```python
from build123d import *

# Parameters (mm, degrees)
F0_W     = 272
F0_H     = 60
F0_R     = 2.75
F0_R_2   = 4
F1_DEPTH = 5


with BuildPart() as f1:
    # F0 (on Front) → F1 (new body)
    with BuildSketch(Plane.XZ):
        Rectangle(F0_W, F0_H)
        with Locations((-62, -12.5)):
            Circle(F0_R, mode=Mode.SUBTRACT)
        with Locations((-16, -12.5)):
            Circle(F0_R, mode=Mode.SUBTRACT)
        with Locations((16, -12.5)):
            Circle(F0_R, mode=Mode.SUBTRACT)
        with Locations((62, -12.5)):
            Circle(F0_R, mode=Mode.SUBTRACT)
        with Locations((-119, 0)):
            Circle(F0_R_2, mode=Mode.SUBTRACT)
        with Locations((-95, 0)):
            Circle(F0_R_2, mode=Mode.SUBTRACT)
        with Locations((-62, 12.5)):
            Circle(F0_R, mode=Mode.SUBTRACT)
        with Locations((-16, 12.5)):
            Circle(F0_R, mode=Mode.SUBTRACT)
        with Locations((16, 12.5)):
            Circle(F0_R, mode=Mode.SUBTRACT)
        with Locations((62, 12.5)):
            Circle(F0_R, mode=Mode.SUBTRACT)
        with Locations((95, 0)):
            Circle(F0_R_2, mode=Mode.SUBTRACT)
        with Locations((119, 0)):
            Circle(F0_R_2, mode=Mode.SUBTRACT)
    extrude(amount=F1_DEPTH)


solid = f1.part
```
The listing builds one solid part. Answer for the finished solid, in the listing's coordinates (mm). Give positions to 0.01 mm unless a question says otherwise; leave off trailing zeros. Order: outer loops, then holes, each group sorted by start corner. A loop starts at its lowest first (then second) coordinate and runs counter-clockwise, first axis right, second up. Notation, with made-up numbers: M 6,63 L 59,63 A23 ccw 59,93 Z; hole C 29,31.5 d11. An arc over 180 degrees is marked long. Put each result on its own line as item: value. Start each with the question number.
Item 1: The part is cut by section D-D, the plane y = -3.85. State how many separate pieces and enclosed holes the cut face has, and give its area (3 significant figures).
Item 2: The part is cut by section A-A, the plane z = 0. Determine the outline of the cut face in (x, y).
Item 3: The part is cut by section C-C, the plane x = 119. Determine the outline of the cut face in (y, z).
Item 4: Find the intervals of material crossed by line 1 along Z through (x, y) = (-16, -1.8); line 2 along Z through (x, y) = (-95, -3); line 3 along X through (y, z) = (-2.55, 14.5), in increasing order.
Item 5: For a pull along Z with two mould halves and no side action, classify faces 1 (the face through (-2, -2, -30)), 2 (the face through (91, -2, 0)), 3 (the face through (136, -2, 0)) as +Z half, -Z half, draft (parallel to the pull), parting line (faces both ways), or undercut.
Item 6: The part is cut by section B-B, the plane x = -62. Determine the outline of the cut face in (y, z).
Answer key:
1. separate pieces: 1
1. enclosed holes: 12
1. area: 15,900 mm²
2. outline: M -136,-5 L -123,-5 L -123,0 L -136,0 Z; M -115,-5 L -99,-5 L -99,0 L -115,0 Z; M -91,-5 L 91,-5 L 91,0 L -91,0 Z; M 99,-5 L 115,-5 L 115,0 L 99,0 Z; M 123,-5 L 136,-5 L 136,0 L 123,0 Z
3. outline: M -5,-30 L 0,-30 L 0,-4 L -5,-4 Z; M -5,4 L 0,4 L 0,30 L -5,30 Z
4. line 1: z = -30 to -15.25, -9.75 to 9.75, 15.25 to 30
4. line 2: z = -30 to -4, 4 to 30
4. line 3: x = -136 to -63.89, -60.11 to -17.89, -14.11 to 14.11, 17.89 to 60.11, 63.89 to 136
5. face 1: -Z half
5. face 2: undercut
5. face 3: draft
6. outline: M -5,-30 L 0,-30 L 0,-15.25 L -5,-15.25 Z; M -5,-9.75 L 0,-9.75 L 0,9.75 L -5,9.75 Z; M -5,15.25 L 0,15.25 L 0,30 L -5,30 Z
